The model under review builds one solid part; all positions refer to its coordinate system, in mm. Face numbers are marked on the shaded views. A direction names the side the tool comes from. Coordinates: 2 decimals unless noted, no trailing zeros. Loops run counter-clockwise (first coordinate to the right, second up) from the corner with the lowest first, then second, coordinate; pieces in that order, holes last. Notation, with made-up numbers: M 78.5,56 L 108.5,56 A21 ccw 108.5,93 Z; hole C -6,-19 d6. An arc over 180 degrees is marked long. Use CSV: the item, a comma, the result in double quotes. Start each with the question number.
1. Add section A-A, the plane x = -20.8. Write out the cut boundary in (y, z), then the cut area to 3 significant figures.
2. Tool access review of the marked faces 5 and 6: name each direction out of +Z, -Z, +X, -X, +Y, -Y from which nothing blocks a thin tool from reaching the whole face with its end or side.
3. Draft analysis for pull direction Y (two halves, no side actions). For the marked faces 1, 2, 3 and 4, state which applies: +Y half, -Y half, draft (parallel to the pull), parting line (faces both ways), or undercut.
4. For L1, parallel to Y at x = 25, z = 1.65; L2, parallel to X at y = -75, z = 2.1; L3, parallel to Y at x = -50, z = 8.25, list the stretches that pass through material, from the lowest coordinate up.
5. Add section C-C, the plane y = -75. Write out the cut boundary in (x, z).
6. Add section D-D, the plane x = 25. Write out the cut boundary in (y, z), then the cut area to 3 significant figures.
7. Add section B-B, the plane z = 12.5. Write out the cut boundary in (x, y).
8. Clearance check with flat-ended pins moving along their axes: P1, Ø3.5, axis at y = 75, z = 12.5, coming from the +X side; P2, Ø2, axis at x = -28, z = 20.5, coming from the -Y side; P3, Ø2.5, axis at y = -75, z = 12.5, coming from the -X side. State where each tip first meets the part, or that it passes through.
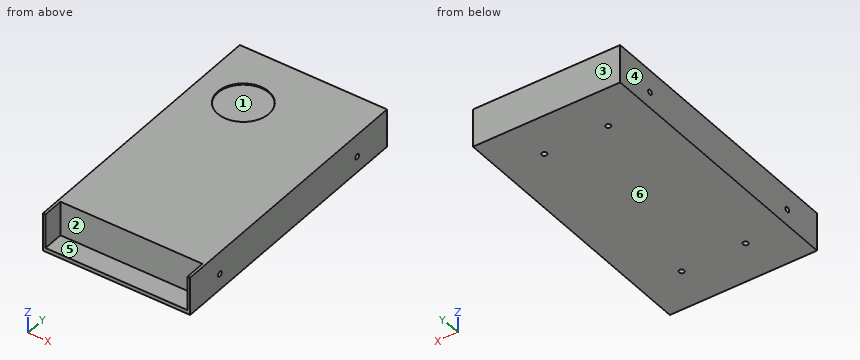
from build123d import *

# Parameters (mm, degrees)
F0_W      = 111
F0_H      = 16.25
F1_DEPTH  = 3
F0_W_2    = 2
F2_DEPTH  = 30
F3_R      = 2
F4_DEPTH  = 5
F5_R      = 2
F6_DEPTH  = 3
F7_R      = 2
F8_DEPTH  = 5
F9_R      = 20
F10_DEPTH = 1


with BuildPart() as f1:
    # F0 (on Top) → F1 (new body)
    with BuildSketch(Plane.XY):
        with Locations((0, -99.375)):
            Rectangle(F0_W, F0_H)
        Polygon((55.5, -91.25), (57.5, -91.25), (57.5, 107.5), (-57.5, 107.5), (-57.5, -91.25), (-55.5, -91.25), align=None)
    extrude(amount=F1_DEPTH)

    # F0 (on Top) → F2 (join)
    with BuildSketch(Plane.XY):
        with Locations((56.5, -99.375)):
            Rectangle(F0_W_2, F0_H)
        with Locations((-56.5, -99.375)):
            Rectangle(F0_W_2, F0_H)
        Polygon((55.5, -91.25), (57.5, -91.25), (57.5, 107.5), (-57.5, 107.5), (-57.5, -91.25), (-55.5, -91.25), align=None)
    extrude(amount=F2_DEPTH)

    # F3 (on face) → F4 (cut)
    with BuildSketch(Plane.YZ.offset(57.5)):
        with Locations((-75, 12.5)):
            Circle(F3_R)
        with Locations((75, 12.5)):
            Circle(F3_R)
    extrude(amount=-F4_DEPTH, mode=Mode.SUBTRACT)

    # F5 (on face) → F6 (cut)
    with BuildSketch(Plane(origin=(0, 0, 0), x_dir=(1, 0, 0), z_dir=(0, 0, -1))):
        with Locations((25, 75)):
            Circle(F5_R)
        with Locations((25, -75)):
            Circle(F5_R)
        with Locations((-25, 75)):
            Circle(F5_R)
        with Locations((-25, -75)):
            Circle(F5_R)
    extrude(amount=-F6_DEPTH, mode=Mode.SUBTRACT)

    # F7 (on face) → F8 (cut)
    with BuildSketch(Plane(origin=(-57.5, 0, 0), x_dir=(0, -1, 0), z_dir=(-1, 0, 0))):
        with Locations((-75, 12.5)):
            Circle(F7_R)
        with Locations((75, 12.5)):
            Circle(F7_R)
    extrude(amount=-F8_DEPTH, mode=Mode.SUBTRACT)

    # F9 (on face) → F10 (cut)
    with BuildSketch(Plane.XY.offset(30)):
        with Locations((-20.8, 60.05)):
            Circle(F9_R)
    extrude(amount=-F10_DEPTH, mode=Mode.SUBTRACT)


solid = f1.part
Computed:
1,outline,"M -107.5,0 L 107.5,0 L 107.5,30 L 80.05,30 L 80.05,29 L 40.05,29 L 40.05,30 L -91.25,30 L -91.25,3 L -107.5,3 Z"
1,area,"5,970 mm^2"
2,face 5,"+Z, -Y"
2,face 6,"-Z, +X, -X, +Y, -Y"
3,face 1,"undercut"
3,face 2,"-Y half"
3,face 3,"+Y half"
3,face 4,"draft"
4,L1,"y = -107.5 to -77, -73 to 73, 77 to 107.5"
4,L2,"x = -57.5 to -27, -23 to 23, 27 to 57.5"
4,L3,"y = -91.25 to 107.5"
5,outline,"M -57.5,0 L -27,0 L -27,3 L -23,3 L -23,0 L 23,0 L 23,3 L 27,3 L 27,0 L 57.5,0 L 57.5,10.5 L 52.5,10.5 L 52.5,14.5 L 57.5,14.5 L 57.5,30 L -57.5,30 L -57.5,14.5 L -52.5,14.5 L -52.5,10.5 L -57.5,10.5 Z"
6,outline,"M -107.5,0 L -77,0 L -77,3 L -73,3 L -73,0 L 73,0 L 73,3 L 77,3 L 77,0 L 107.5,0 L 107.5,30 L -91.25,30 L -91.25,3 L -107.5,3 Z"
6,area,"5,990 mm^2"
7,outline,"M -57.5,-107.5 L -55.5,-107.5 L -55.5,-91.25 L 55.5,-91.25 L 55.5,-107.5 L 57.5,-107.5 L 57.5,-77 L 52.5,-77 L 52.5,-73 L 57.5,-73 L 57.5,73 L 52.5,73 L 52.5,77 L 57.5,77 L 57.5,107.5 L -57.5,107.5 L -57.5,77 L -52.5,77 L -52.5,73 L -57.5,73 L -57.5,-73 L -52.5,-73 L -52.5,-77 L -57.5,-77 Z"
8,P1,"stops at x = 52.5"
8,P2,"stops at y = -91.25"
8,P3,"stops at x = -52.5"
